Part model, mm, in its own coordinate system. A direction names the side the tool comes from. Coordinates: 2 decimals unless noted, no trailing zeros. Loops run counter-clockwise (first coordinate to the right, second up) from the corner with the lowest first, then second, coordinate; pieces in that order, holes last. Notation, with made-up numbers: (64.5, -38) - (81.5, -38) arc R8 ccw to (81.5, -23) - close; hole circle Ø3 at (26, -13.75). An arc over 180 degrees is marked (long way). One line per question, with ' | ' between items. Start each with the question number.
from build123d import *

# Parameters (mm, degrees)
SKETCH1_W           = 2.5
SKETCH1_H           = 22.5
BOSS_EXTRUDE1_DEPTH = 14
CUT_EXTRUDE2_DEPTH  = 23.25
SKETCH6_R           = 2.25
CUT_EXTRUDE3_DEPTH  = 75.434954826
SKETCH7_R           = 50
SKETCH7_R_2         = 12.65
CUT_EXTRUDE6_DEPTH  = 74.284121745


with BuildPart() as part:
    # Sketch1 → Revolve1 (revolve)
    with BuildSketch(Plane.XY, mode=Mode.PRIVATE) as revolve1_sk:
        Polygon((0, 12.65), (0, 0), (19.25, 0), (19.25, 9.144072085), (9.207200807, 18.137623601), (-1.247452839, 27.5), (-3, 27.5), (-3, 12.65), align=None)
        with BuildLine():
            Line((-1.247452839, 27.5), (9.207200807, 18.137623601))
            ThreePointArc((9.207200807, 18.137623601), (5.339394973, 22.45043534), (2.5, 27.5))
            Line((2.5, 27.5), (0, 27.5))
            Line((0, 27.5), (-1.247452839, 27.5))
        make_face()
        with BuildLine():
            Line((9.207200807, 18.137623601), (19.25, 9.144072085))
            Line((19.25, 9.144072085), (19.25, 12.5))
            ThreePointArc((19.25, 12.5), (13.918967856, 14.767235866), (9.207200807, 18.137623601))
        make_face()
        with Locations((1.25, 38.75)):
            Rectangle(SKETCH1_W, SKETCH1_H)
    revolve(revolve1_sk.sketch.rotate(Axis((-75.117650177, 0, 0), (1, 0, 0)), 90), axis=Axis((-75.117650177, 0, 0), (1, 0, 0)))

    # Sketch3 → Boss-Extrude1 (add)
    with BuildSketch(Plane.ZY):
        with BuildLine():
            Line((-2.4, 8.8), (-2.4, 6.469157596))
            ThreePointArc((-2.4, 6.469157596), (0, 6.9), (2.4, 6.469157596))
            Line((2.4, 6.469157596), (2.4, 8.8))
            Line((2.4, 8.8), (-2.4, 8.8))
        make_face()
        with BuildLine():
            Line((-2.4, 6.469157596), (-2.4, 0))
            Line((-2.4, 0), (2.4, 0))
            Line((2.4, 0), (2.4, 6.469157596))
            ThreePointArc((2.4, 6.469157596), (0, 6.9), (-2.4, 6.469157596))
        make_face()
        with BuildLine():
            Line((2.4, 0), (-2.4, 0))
            Line((-2.4, 0), (-2.4, 6.469157596))
            ThreePointArc((-2.4, 6.469157596), (-3.940177661, -5.664362277), (6.9, 0))
            ThreePointArc((6.9, 0), (5.664362277, 3.940177661), (2.4, 6.469157596))
            Line((2.4, 6.469157596), (2.4, 0))
        make_face()
    extrude(amount=BOSS_EXTRUDE1_DEPTH)

    # Sketch5 → Cut-Extrude2 (cut)
    with BuildSketch(Plane(origin=(19.25, 0, 0), x_dir=(0, 0, -1), z_dir=(1, 0, 0))):
        with BuildLine():
            Line((2.25, 7.8), (-2.25, 7.8))
            Line((-2.25, 7.8), (-2.25, 5.830951895))
            ThreePointArc((-2.25, 5.830951895), (0, 6.25), (2.25, 5.830951895))
            Line((2.25, 5.830951895), (2.25, 7.8))
        make_face()
        with BuildLine():
            ThreePointArc((2.25, 5.830951895), (0, 6.25), (-2.25, 5.830951895))
            Line((-2.25, 5.830951895), (-2.25, 0))
            Line((-2.25, 0), (2.25, 0))
            Line((2.25, 0), (2.25, 5.830951895))
        make_face()
        with BuildLine():
            Line((-2.25, 0), (-2.25, 5.830951895))
            ThreePointArc((-2.25, 5.830951895), (-3.535533906, -5.153882032), (6.25, 0))
            ThreePointArc((6.25, 0), (5.153882032, 3.535533906), (2.25, 5.830951895))
            Line((2.25, 5.830951895), (2.25, 0))
            Line((2.25, 0), (-2.25, 0))
        make_face()
    extrude(amount=-CUT_EXTRUDE2_DEPTH, mode=Mode.SUBTRACT)

    # Sketch6 → Cut-Extrude3 (cut, through all)
    with BuildSketch(Plane(origin=(-4, 0, 0), x_dir=(0, 0, -1), z_dir=(1, 0, 0))):
        Circle(SKETCH6_R)
    extrude(amount=-CUT_EXTRUDE3_DEPTH, mode=Mode.SUBTRACT)

    # Sketch7 → Cut-Extrude6 (cut, through all)
    with BuildSketch(Plane.ZY):
        Circle(SKETCH7_R)
        Circle(SKETCH7_R_2, mode=Mode.SUBTRACT)
    extrude(amount=CUT_EXTRUDE6_DEPTH, mode=Mode.SUBTRACT)


solid = part.part
1) Band-saw the part on C-C on y = 37.5. List the corners of the cut face in (x, z).
2) Band-saw the part on D-D on y = -37. List the corners of the cut face in (x, z).
3) Band-saw the part on B-B on x = 7. List the corners of the cut face in (y, z).
4) Wall check: line 1 along Y through (x, z) = (-10, 0); line 2 along X through (y, z) = (37.5, -21.5); line 3 along Y through (x, z) = (6, 0). Give the ranges that are in metal, low to high. Write a range as [from, to].
5) Pin check, flat tips, straight feed: pin 1 Ø1.9 at (x, y) = (-7, 8) entering from -Z; pin 2 Ø5 at (x, z) = (3, 0) entering from -Y; pin 3 Ø2.5 at (x, z) = (-6, 1) entering from +Y; pin 4 Ø12 at (x, y) = (-8.5, 34) entering from -Z. Stop position of each tip, or through.
6) Mould opens along Z. For faces 5 (the cylindrical face through (-8.93, 2.23, 0.29)), 6 (the flat face through (8, 7.8, 0)), 7 (the flat face through (2.5, 22, -22)), 8 (the flat face through (-7, 8, 2.4)) say: +Z half, -Z half, draft (parallel to the pull), parting line (faces both ways), or undercut.
7) Band-saw the part on A-A on x = -6.5. List the corners of the cut face in (y, z).
8) Tool access for faces 1 (the flat face through (-7, 8.8, 0)), 2 (the flat face through (-4, 2.4, 0.1)), 3 (the flat face through (-7, 8, -2.4)), 4 (the flat face through (-14, 3, 0)): list every direction of +Z, -Z, +X, -X, +Y, -Y with a clear straight run to the whole face (end or side of a thin tool).
Values found:
1) outline: (0, -33.07) - (2.5, -33.07) - (2.5, 33.07) - (0, 33.07) - close
2) outline: (0, -33.63) - (2.5, -33.63) - (2.5, 33.63) - (0, 33.63) - close
3) outline: circle Ø40.73 at (0, 0); hole (5.83, -2.25) - (7.8, -2.25) - (7.8, 2.25) - (5.83, 2.25) arc R6.25 ccw (long way) to start
4) line 1: [-6.9, -2.25], [2.25, 8.8] | line 2: [0, 2.5] | line 3: [-21.57, -6.25], [7.8, 21.57]
5) pin 1: z = -2.4 | pin 2: y = -50 | pin 3: y = 8.8 | pin 4: through
6) face 5: undercut | face 6: undercut | face 7: draft | face 8: +Z half
7) outline: (6.47, -2.4) - (8.8, -2.4) - (8.8, 2.4) - (6.47, 2.4) arc R6.9 ccw (long way) to start; hole circle Ø4.5 at (0, 0)
8) face 1: +Z, -Z, -X, +Y | face 2: +X | face 3: -Z, -X, +Y | face 4: +Z, -Z, -X, +Y, -Y
